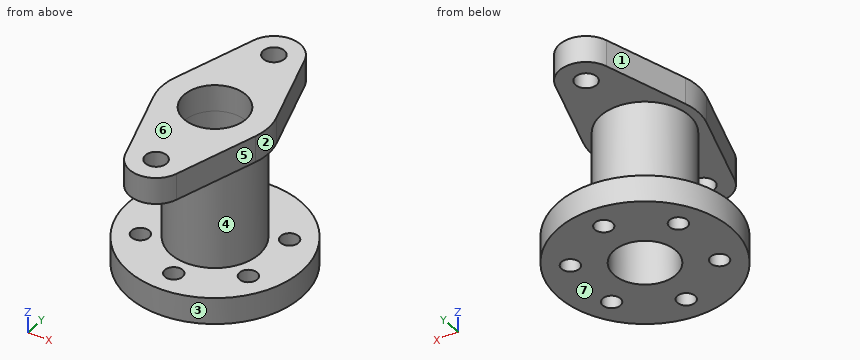
```python
from build123d import *

# Parameters (mm, degrees)
SKETCH2_R           = 6
SKETCH2_R_2         = 17.5
BOSS_EXTRUDE1_DEPTH = 15
SKETCH3_R           = 25
BOSS_EXTRUDE3_DEPTH = 60
SKETCH4_R           = 49
BOSS_EXTRUDE4_DEPTH = 15
SKETCH5_R           = 5
CUT_EXTRUDE1_DEPTH  = 15
SKETCH6_R           = 17.5
CUT_EXTRUDE2_DEPTH  = 111.684235553


with BuildPart() as part:
    # Sketch2 → Boss-Extrude1 (new body)
    with BuildSketch(Plane.XY):
        with BuildLine():
            Line((14.309088021, 54.5), (28.618176043, 9))
            ThreePointArc((28.618176043, 9), (30, 0), (28.618176043, -9))
            Line((28.618176043, -9), (14.309088021, -54.5))
            ThreePointArc((14.309088021, -54.5), (0, -65), (-14.309088021, -54.5))
            Line((-14.309088021, -54.5), (-28.618176043, -9))
            ThreePointArc((-28.618176043, -9), (-30, 0), (-28.618176043, 9))
            Line((-28.618176043, 9), (-14.309088021, 54.5))
            ThreePointArc((-14.309088021, 54.5), (0, 65), (14.309088021, 54.5))
        make_face()
        with Locations((0, 50)):
            Circle(SKETCH2_R, mode=Mode.SUBTRACT)
        Circle(SKETCH2_R_2, mode=Mode.SUBTRACT)
        with Locations(Location((0, -50, 0), (0, 0, 180))):
            Circle(SKETCH2_R, mode=Mode.SUBTRACT)
    extrude(amount=BOSS_EXTRUDE1_DEPTH)

    # Sketch3 → Boss-Extrude3 (add)
    with BuildSketch(Plane(origin=(0, 0, 0), x_dir=(-1, 0, 0), z_dir=(0, 0, -1))):
        with Locations(Location((0, 0, 0), (0, 0, 180))):
            Circle(SKETCH3_R)
    extrude(amount=BOSS_EXTRUDE3_DEPTH)

    # Sketch4 → Boss-Extrude4 (add)
    with BuildSketch(Plane(origin=(0, 0, -60), x_dir=(-1, 0, 0), z_dir=(0, 0, -1))):
        Circle(SKETCH4_R)
    extrude(amount=BOSS_EXTRUDE4_DEPTH)

    # Sketch5 → Cut-Extrude1 (cut)
    with BuildSketch(Plane(origin=(0, 0, -75), x_dir=(-1, 0, 0), z_dir=(0, 0, -1))):
        with Locations((0, 35)):
            Circle(SKETCH5_R)
        with Locations((30.310889132, 17.5)):
            Circle(SKETCH5_R)
        with Locations((30.310889132, -17.5)):
            Circle(SKETCH5_R)
        with Locations((0, -35)):
            Circle(SKETCH5_R)
        with Locations((-30.310889132, -17.5)):
            Circle(SKETCH5_R)
        with Locations((-30.310889132, 17.5)):
            Circle(SKETCH5_R)
    extrude(amount=-CUT_EXTRUDE1_DEPTH, mode=Mode.SUBTRACT)

    # Sketch6 → Cut-Extrude2 (cut, through all)
    with BuildSketch(Plane.XY):
        Circle(SKETCH6_R)
    extrude(amount=-CUT_EXTRUDE2_DEPTH, mode=Mode.SUBTRACT)


solid = part.part
```
Read the model definition and answer for the solid it produces. Units are mm, in the model's axes. Face numbers are marked on the shaded views. A direction names the side the tool comes from. Give positions to 0.01 mm unless a question says otherwise; leave off trailing zeros. Order: outer loops, then holes, each group sorted by start corner. A loop starts at its lowest first (then second) coordinate and runs counter-clockwise, first axis right, second up. Notation, with made-up numbers: (15.25, 60) -> (54.25, 60) arc R16 ccw to (54.25, 68) -> close; hole circle Ø10 at (49.5, -24). An arc over 180 degrees is marked (long way). One line per item, written item: value. Start each with the question number.
(1) The part is cut by section B-B (x = 0). State how many separate pieces and enclosed holes the cut face has, and give its area (3 significant figures).
(2) The part is cut by section C-C (z = 4). Determine the outline of the cut face in (x, y), and give its area (3 significant figures).
(3) A tool of negligible diameter and unlimited length cuts with its end or side. For the marked faces 1, 2 and 3, from which of +Z, -Z, +X, -X, +Y, -Y can it reach the whole face along a straight path? Write none if from no direction.
(4) Straight lines are drawn through the part: L1, parallel to Y at x = 0, z = 3.75; L2, parallel to Y at x = 0, z = -65; L3, parallel to Z at x = -14, y = 45. For each, find the intervals that lie inside material, in ascending order.
(5) For a pull along Z with two mould halves and no side action, classify the marked faces 4, 5, 6 and 7 as released by +Z, released by -Z, zero draft, split by the parting line, or undercut.
(6) Flat-ended cylindrical pins translate along their axes: P1, Ø10, axis at y = -30.5, z = -36, coming from the -X side; P2, Ø9.5, axis at x = 0, y = 50, coming from the +Z side; P3, Ø6, axis at x = 0, y = -35, coming from the -Z side; P4, Ø6, axis at x = -15.5, z = -45.5, coming from the +Y side. Find the tip coordinate at first contact, or state that the pin passes through.
(7) The part is cut by section D-D (y = -14). Determine the outline of the cut face in (x, z).
(8) The part is cut by section A-A (y = 0). Determine the outline of the cut face in (x, z), and give its area (3 significant figures).
Taken from the geometry:
1. separate pieces: 6
1. enclosed holes: 0
1. area: 2,610 mm^2
2. outline: (-28.62, -9) -> (-14.31, -54.5) arc R15 ccw to (14.31, -54.5) -> (28.62, -9) arc R30 ccw to (28.62, 9) -> (14.31, 54.5) arc R15 ccw to (-14.31, 54.5) -> (-28.62, 9) arc R30 ccw to start; hole circle Ø35 at (0, 0); hole circle Ø12 at (0, -50); hole circle Ø12 at (0, 50)
2. area: 4,220 mm^2
3. face 1: +Z, -X, +Y
3. face 2: +Z, +X
3. face 3: -Z
4. L1: -65 to -56, -44 to -17.5, 17.5 to 44, 56 to 65
4. L2: -49 to -40, -30 to -17.5, 17.5 to 30, 40 to 49
4. L3: -75 to -60, 0 to 15
5. face 4: undercut
5. face 5: zero draft
5. face 6: released by +Z
5. face 7: released by -Z
6. P1: through
6. P2: z = -60
6. P3: z = 0
6. P4: y = 21.65
7. outline: (-46.96, -75) -> (-33.88, -75) -> (-33.88, -60) -> (-46.96, -60) -> close; (-27.05, 0) -> (-20.71, 0) -> (-20.71, -60) -> (-26.74, -60) -> (-26.74, -75) -> (-10.5, -75) -> (-10.5, 15) -> (-27.05, 15) -> close; (10.5, -75) -> (26.74, -75) -> (26.74, -60) -> (20.71, -60) -> (20.71, 0) -> (27.05, 0) -> (27.05, 15) -> (10.5, 15) -> close; (33.88, -75) -> (46.96, -75) -> (46.96, -60) -> (33.88, -60) -> close
8. outline: (-49, -75) -> (-17.5, -75) -> (-17.5, 15) -> (-30, 15) -> (-30, 0) -> (-25, 0) -> (-25, -60) -> (-49, -60) -> close; (17.5, -75) -> (49, -75) -> (49, -60) -> (25, -60) -> (25, 0) -> (30, 0) -> (30, 15) -> (17.5, 15) -> close
8. area: 2,220 mm^2
